from build123d import *

# Parameters (mm, degrees)
F0_R          = 11.1125
F1_DEPTH      = 152.4
F2_SIZE       = 3.175
F3_R          = 4.7625
F4_DEPTH      = 25.4
F4_DEPTH_BACK = 25.4
F5_R          = 3.175
F6_DEPTH      = 12.7


with BuildPart() as f1:
    # F0 (on Top) → F1 (new body)
    with BuildSketch(Plane.XY):
        with Locations((-1.1552e-06, 0.1656521781)):
            Circle(F0_R)
    extrude(amount=F1_DEPTH)

    # F2
    f2_edges = [f1.edges().sort_by_distance(p)[0] for p in [
        (-11.112501, 0.165652, 0),
    ]]
    chamfer(f2_edges, length=F2_SIZE)

    # F3 (on Front) → F4 (cut, two sides)
    with BuildSketch(Plane.XZ) as f4_sk:
        with Locations((0, 133.35)):
            Circle(F3_R)
    extrude(amount=-F4_DEPTH, mode=Mode.SUBTRACT)
    extrude(f4_sk.sketch, amount=F4_DEPTH_BACK, mode=Mode.SUBTRACT)

    # F5 (on face) → F6 (cut)
    with BuildSketch(Plane.XY.offset(152.4)):
        Circle(F5_R)
    extrude(amount=-F6_DEPTH, mode=Mode.SUBTRACT)


solid = f1.part
Design review of the part built by this model. Coordinates are the model's own, in mm. A direction names the side the tool comes from. Round coordinates to 2 decimals unless told otherwise and drop trailing zeros. Order: outer loops, then holes, each group sorted by start corner. A loop starts at its lowest first (then second) coordinate and runs counter-clockwise, first axis right, second up.
1) Consider section B-B (z = 68). State the section outline as (x, y) points (1 decimal), plus the area to 3 significant figures.
The answers:
outline: circle Ø22.2 at (0, 0.2)
area: 388 mm2
2) Consider section A-A (z = 133.35). State the section outline as (x, y) points (1 decimal), plus the area to 3 significant figures.
The answers:
outline: (-4.8, -9.9) - (-4.8, 10.2) arc R11.1 ccw to start; (4.8, -9.9) arc R11.1 ccw to (4.8, 10.2) - close
area: 183 mm2
3) Clearance check with flat-ended pins moving along their axes: pin 1 Ø1 at (x, z) = (7.5, 45.5) entering from +Y; pin 2 Ø2 at (y, z) = (5.5, 78) entering from +X; pin 3 Ø5.5 at (x, z) = (0, 133.35) entering from +Y; pin 4 Ø2 at (x, z) = (-3, 88) entering from +Y. State where each tip first meets the part, or that it passes through.
The answers:
pin 1: stops at y = 8.8
pin 2: stops at x = 10.23
pin 3: passes through
pin 4: stops at y = 11.1
4) Machinability: for faces 1 (the cylindrical face through (10.6, 3.5, 76.7)), 2 (the flat face through (0, 0, 139.7)), which of the approach directions +Z, -Z, +X, -X, +Y, -Y give a long, thin tool a straight path to every point of the face, cutting with its end or side? Answer none if there is none.
The answers:
face 1: +Z, -Z
face 2: +Z
5) For L1, parallel to Y at x = 0, z = 146 (3 decimals); L2, parallel to Z at x = 0, y = -2.5; L3, parallel to Z at x = 0, y = 6.5, list the stretches that pass through material, from the lowest coordinate up.
The answers:
L1: y = -10.947 to -3.175, 3.175 to 11.278
L2: z = 0 to 128.59, 138.11 to 139.7
L3: z = 0 to 128.59, 138.11 to 152.4
6) Draft analysis for pull direction X (two halves, no side actions). For faces 3 (the cylindrical face through (-1.03, 0.01, 128.7)), 4 (the flat face through (-3, -2, 152.4)), 5 (the conical face through (7.718, 2.596, 0.154)), state which applies: released by +X, released by -X, zero draft, split by the parting line, or undercut.
The answers:
face 3: undercut
face 4: zero draft
face 5: split by the parting line
